Can you work these out from the model? Positions are in its coordinate system, mm. Face numbers are marked on the shaded views. A direction names the side the tool comes from. Coordinates: 2 decimals unless noted, no trailing zeros. Write each loop counter-clockwise with the first axis right and the second up, starting at its lowest first coordinate (ties: lowest second). Pieces come first, ordered by that corner, then holes. Notation, with made-up numbers: (-40, 37) - (-24, 37) arc R31 cw to (-24, 72) - close; hole circle Ø4 at (-29.5, 11.25). An arc over 180 degrees is marked (long way). Use one line per item in the form item = value. Start each with the question number.
(1) On a 3-axis mill with a long thin cutter (end or side, diameter ignored), from which of +Z, -Z, +X, -X, +Y, -Y can I reach the whole of each face in a straight line? I mean the marked faces 1, 2, 3 and 4. Say none if no direction works.
(2) If I drill on probe 1 along Y at (x, z) = (-56.5, -13.5); probe 2 along X at (y, z) = (-3.5, 15.5), over which ranges is the centre line in solid material (lowest first)? Write a range as from..to.
(3) If we section it at C-C on x = -57.5: Please give me the cut outline in (y, z), then the cut area to 3 significant figures.
(4) If we section it at A-A on y = -2.5: Please give me the cut outline in (x, z).
(5) If we section it at B-B on z = 13.5: Please give me the cut outline in (x, y), then the cut area to 3 significant figures.
(6) For pin 1 Ø1 at (x, y) = (-58.5, -9) entering from +Z; pin 2 Ø1.6 at (x, y) = (-56.5, 0.5) entering from +Z; pin 3 Ø3 at (y, z) = (3, -17) entering from +X, each with a flat end and sliding along its axis, tell me the tip position at first contact or that it passes through.
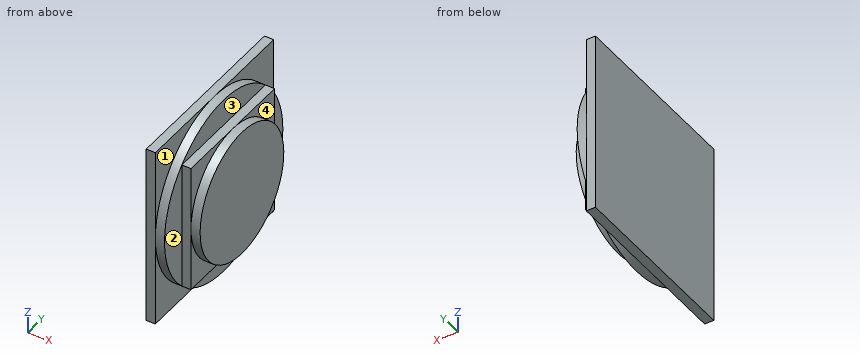
```python
from build123d import *

# Parameters (mm, degrees)
F0_W     = 2
F0_H     = 40
F1_DEPTH = 20
F2_W     = 2
F2_H     = 20
F5_W     = 28.284272
F5_H     = 28.284272
F6_DEPTH = 2
F7_W     = 2
F7_H     = 14.142136


with BuildPart() as f1:
    # F0 (on Front) → F1 (new body, symmetric)
    with BuildSketch(Plane.XZ):
        with Locations((-61, 0)):
            Rectangle(F0_W, F0_H)
    extrude(amount=F1_DEPTH, both=True)

    # F2 (on Front) → F3 (revolve)
    with BuildSketch(Plane.XZ):
        with Locations((-59, 10)):
            Rectangle(F2_W, F2_H)
    revolve(axis=Axis((-60, 0, 0), (-1, 0, 0)))

    # F5 (on offset) → F6 (join)
    with BuildSketch(Plane.YZ.offset(-58)):
        Rectangle(F5_W, F5_H)
    extrude(amount=F6_DEPTH)

    # F7 (on Front) → F8 (revolve)
    with BuildSketch(Plane.XZ):
        with Locations((-55, 7.071068)):
            Rectangle(F7_W, F7_H)
    revolve(axis=Axis((-55, 0, 0), (-1, 0, 0)))


solid = f1.part
```
Reported:
q1.face_1 = +Z, +X, -Y
q1.face_2 = +Z, -Z, +X, -Y
q1.face_3 = +Z, +X, +Y, -Y
q1.face_4 = +Z, +X, +Y
q2.probe_1 = -14.14..14.14
q2.probe_2 = -62..-58
q3.outline = (-14.14, -14.14) - (14.14, -14.14) - (14.14, 14.14) - (-14.14, 14.14) - close
q3.area = 800 mm2
q4.outline = (-62, -20) - (-60, -20) - (-60, -19.84) - (-58, -19.84) - (-58, -14.14) - (-56, -14.14) - (-56, -13.92) - (-54, -13.92) - (-54, 13.92) - (-56, 13.92) - (-56, 14.14) - (-58, 14.14) - (-58, 19.84) - (-60, 19.84) - (-60, 20) - (-62, 20) - close
q5.outline = (-62, -20) - (-60, -20) - (-60, -14.76) - (-58, -14.76) - (-58, -14.14) - (-56, -14.14) - (-56, -4.21) - (-54, -4.21) - (-54, 4.21) - (-56, 4.21) - (-56, 14.14) - (-58, 14.14) - (-58, 14.76) - (-60, 14.76) - (-60, 20) - (-62, 20) - close
q5.area = 212 mm2
q6.pin_1 = 18.1
q6.pin_2 = 14.14
q6.pin_3 = -58
